Read the model definition and answer for the solid it produces. Units are mm, in the model's axes. A direction names the side the tool comes from. Coordinates: 2 decimals unless noted, no trailing zeros. Loops run counter-clockwise (first coordinate to the right, second up) from the corner with the lowest first, then second, coordinate; pieces in that order, holes last.
from build123d import *

# Parameters (mm, degrees)
SKETCH1_W                             = 70
SKETCH1_H                             = 110
BOTTOM_DEPTH                          = 3.5
SKETCH3_W                             = 70
SKETCH3_H                             = 110
WALL_DEPTH                            = 40
SKETCH4_R                             = 1.625
TOP_PLATE_SCREW_HOLES_DEPTH           = 30
TOP_PLATE_SCREW_HOLES_DRAFT           = -1
TOP_PLATE_SCREW_HOLES_PROFILE_2_DEPTH = 30
TOP_PLATE_SCREW_HOLES_PROFILE_2_DRAFT = -1
TOP_PLATE_SCREW_HOLES_PROFILE_3_DEPTH = 30
TOP_PLATE_SCREW_HOLES_PROFILE_3_DRAFT = -1
TOP_PLATE_SCREW_HOLES_PROFILE_4_DEPTH = 30
TOP_PLATE_SCREW_HOLES_PROFILE_4_DRAFT = -1
FILLET1_R                             = 2
FILLET2_R                             = 2
FILLET3_R                             = 2
FILLET4_R                             = 2
FILLET5_R                             = 2
FILLET6_R                             = 2
FILLET7_R                             = 2
FILLET8_R                             = 2
M4_MOUNT_R                            = 2.1
M4_MOUNT_CUT_DEPTH                    = 77.485292704
CABLE_PASS_CUT_DEPTH                  = 10
SKETCH6_R                             = 1.75
M3_CONNECTION_CUT_DEPTH               = 10


with BuildPart() as part:
    # Sketch1 → Bottom (new body)
    with BuildSketch(Plane(origin=(0, 0, 0), x_dir=(1, 0, 0), z_dir=(0, 1, 0))):
        Rectangle(SKETCH1_W, SKETCH1_H)
    extrude(amount=BOTTOM_DEPTH)

    # Sketch3 → Wall (add)
    with BuildSketch(Plane(origin=(0, 3.5, 0), x_dir=(1, 0, 0), z_dir=(0, 1, 0))):
        Rectangle(SKETCH3_W, SKETCH3_H)
        Polygon((-26, 52), (-4, 52), (26, 52), (26, 46), (32, 46), (32, -46), (26, -46), (26, -52), (4, -52), (-26, -52), (-26, -46), (-32, -46), (-32, 46), (-26, 46), align=None, mode=Mode.SUBTRACT)
    extrude(amount=WALL_DEPTH)


with BuildPart() as top_plate_screw_holes_tool:
    # Sketch4 → Top Plate Screw Holes (with draft: the straight prism first)
    with BuildSketch(Plane(origin=(0, 43.5, 0), x_dir=(1, 0, 0), z_dir=(0, 1, 0))):
        with Locations((-30, 50)):
            Circle(SKETCH4_R)
    extrude(amount=-TOP_PLATE_SCREW_HOLES_DEPTH)
    # Top Plate Screw Holes: the draft: its side faces are tilted about the plane it starts from
    top_plate_screw_holes_sides = [top_plate_screw_holes_tool.faces().sort_by_distance(p)[0] for p in [
        (-31.625, 28.5, -50),
    ]]
    draft(top_plate_screw_holes_sides, Plane(origin=(0, 43.5, 0), x_dir=(1, 0, 0), z_dir=(0, 1, 0)), TOP_PLATE_SCREW_HOLES_DRAFT)


with BuildPart() as part_1:
    add(part.part)

    # Top Plate Screw Holes: cut by top_plate_screw_holes_tool
    add(top_plate_screw_holes_tool.part, mode=Mode.SUBTRACT)


with BuildPart() as top_plate_screw_holes_profile_2_tool:
    # Sketch4 → Top Plate Screw Holes profile 2 (with draft: the straight prism first)
    with BuildSketch(Plane(origin=(0, 43.5, 0), x_dir=(1, 0, 0), z_dir=(0, 1, 0))):
        with Locations((30, 50)):
            Circle(SKETCH4_R)
    extrude(amount=-TOP_PLATE_SCREW_HOLES_PROFILE_2_DEPTH)
    # Top Plate Screw Holes profile 2: the draft: its side faces are tilted about the plane it starts from
    top_plate_screw_holes_profile_2_sides = [top_plate_screw_holes_profile_2_tool.faces().sort_by_distance(p)[0] for p in [
        (28.375, 28.5, -50),
    ]]
    draft(top_plate_screw_holes_profile_2_sides, Plane(origin=(0, 43.5, 0), x_dir=(1, 0, 0), z_dir=(0, 1, 0)), TOP_PLATE_SCREW_HOLES_PROFILE_2_DRAFT)


with BuildPart() as part_2:
    add(part_1.part)

    # Top Plate Screw Holes profile 2: cut by top_plate_screw_holes_profile_2_tool
    add(top_plate_screw_holes_profile_2_tool.part, mode=Mode.SUBTRACT)


with BuildPart() as top_plate_screw_holes_profile_3_tool:
    # Sketch4 → Top Plate Screw Holes profile 3 (with draft: the straight prism first)
    with BuildSketch(Plane(origin=(0, 43.5, 0), x_dir=(1, 0, 0), z_dir=(0, 1, 0))):
        with Locations((30, -50)):
            Circle(SKETCH4_R)
    extrude(amount=-TOP_PLATE_SCREW_HOLES_PROFILE_3_DEPTH)
    # Top Plate Screw Holes profile 3: the draft: its side faces are tilted about the plane it starts from
    top_plate_screw_holes_profile_3_sides = [top_plate_screw_holes_profile_3_tool.faces().sort_by_distance(p)[0] for p in [
        (28.375, 28.5, 50),
    ]]
    draft(top_plate_screw_holes_profile_3_sides, Plane(origin=(0, 43.5, 0), x_dir=(1, 0, 0), z_dir=(0, 1, 0)), TOP_PLATE_SCREW_HOLES_PROFILE_3_DRAFT)


with BuildPart() as part_3:
    add(part_2.part)

    # Top Plate Screw Holes profile 3: cut by top_plate_screw_holes_profile_3_tool
    add(top_plate_screw_holes_profile_3_tool.part, mode=Mode.SUBTRACT)


with BuildPart() as top_plate_screw_holes_profile_4_tool:
    # Sketch4 → Top Plate Screw Holes profile 4 (with draft: the straight prism first)
    with BuildSketch(Plane(origin=(0, 43.5, 0), x_dir=(1, 0, 0), z_dir=(0, 1, 0))):
        with Locations((-30, -50)):
            Circle(SKETCH4_R)
    extrude(amount=-TOP_PLATE_SCREW_HOLES_PROFILE_4_DEPTH)
    # Top Plate Screw Holes profile 4: the draft: its side faces are tilted about the plane it starts from
    top_plate_screw_holes_profile_4_sides = [top_plate_screw_holes_profile_4_tool.faces().sort_by_distance(p)[0] for p in [
        (-31.625, 28.5, 50),
    ]]
    draft(top_plate_screw_holes_profile_4_sides, Plane(origin=(0, 43.5, 0), x_dir=(1, 0, 0), z_dir=(0, 1, 0)), TOP_PLATE_SCREW_HOLES_PROFILE_4_DRAFT)


with BuildPart() as part_4:
    add(part_3.part)

    # Top Plate Screw Holes profile 4: cut by top_plate_screw_holes_profile_4_tool
    add(top_plate_screw_holes_profile_4_tool.part, mode=Mode.SUBTRACT)

    # Fillet1
    fillet1_edges = [part_4.edges().sort_by_distance(p)[0] for p in [
        (-26, 23.5, 46),
    ]]
    fillet(fillet1_edges, radius=FILLET1_R)

    # Fillet2
    fillet2_edges = [part_4.edges().sort_by_distance(p)[0] for p in [
        (26, 23.5, 46),
    ]]
    fillet(fillet2_edges, radius=FILLET2_R)

    # Fillet3
    fillet3_edges = [part_4.edges().sort_by_distance(p)[0] for p in [
        (26, 23.5, -46),
    ]]
    fillet(fillet3_edges, radius=FILLET3_R)

    # Fillet4
    fillet4_edges = [part_4.edges().sort_by_distance(p)[0] for p in [
        (-26, 23.5, -46),
    ]]
    fillet(fillet4_edges, radius=FILLET4_R)

    # Fillet5
    fillet5_edges = [part_4.edges().sort_by_distance(p)[0] for p in [
        (-35, 21.75, -55),
    ]]
    fillet(fillet5_edges, radius=FILLET5_R)

    # Fillet6
    fillet6_edges = [part_4.edges().sort_by_distance(p)[0] for p in [
        (35, 21.75, -55),
    ]]
    fillet(fillet6_edges, radius=FILLET6_R)

    # Fillet7
    fillet7_edges = [part_4.edges().sort_by_distance(p)[0] for p in [
        (35, 21.75, 55),
    ]]
    fillet(fillet7_edges, radius=FILLET7_R)

    # Fillet8
    fillet8_edges = [part_4.edges().sort_by_distance(p)[0] for p in [
        (-35, 21.75, 55),
    ]]
    fillet(fillet8_edges, radius=FILLET8_R)

    # M4 Mount → M4 Mount Cut (cut, through all)
    with BuildSketch(Plane.XZ.offset(-3.5)):
        with Locations(Location((0, -20, 0), (0, 0, 270))):
            Circle(M4_MOUNT_R)
        with Locations(Location((0, 20, 0), (0, 0, 270))):
            Circle(M4_MOUNT_R)
    extrude(amount=M4_MOUNT_CUT_DEPTH, mode=Mode.SUBTRACT)

    # M4 Screw CUT cone 1 section (through the dimple's axis) → M4 Screw CUT (revolve, cut)
    with BuildSketch(Plane(origin=(0, 3.5, 20), x_dir=(0, 0, 1), z_dir=(1, 0, 0))):
        Polygon((0, 0), (3.75, 0), (0, 3.75), align=None)
    revolve(axis=Axis((0, 3.5, 20), (0, -1, 0)), mode=Mode.SUBTRACT)

    # M4 Screw CUT cone 2 section (through the dimple's axis) → M4 Screw CUT cone 2 (revolve, cut)
    with BuildSketch(Plane(origin=(0, 3.5, -20), x_dir=(0, 0, 1), z_dir=(1, 0, 0))):
        Polygon((0, 0), (3.75, 0), (0, 3.75), align=None)
    revolve(axis=Axis((0, 3.5, -20), (0, -1, 0)), mode=Mode.SUBTRACT)

    # Sketch5 → Cable Pass CUT (cut)
    with BuildSketch(Plane.ZY.offset(-32)):
        with BuildLine():
            Line((-46, 3.5), (-34, 3.5))
            add(Edge.make_bspline(
                [(-34, 3.5), (-34, 6.5), (-40, 6.5), (-46, 6.5), (-46, 3.5)],
                knots=[0, 0, 0, 1.570796327, 1.570796327, 3.141592654, 3.141592654, 3.141592654], degree=2, weights=[1, 0.707106781, 1, 0.707106781, 1]))
        make_face()
    extrude(amount=-CABLE_PASS_CUT_DEPTH, mode=Mode.SUBTRACT)

    # Sketch6 → M3 Connection CUT (cut)
    with BuildSketch(Plane.ZY.offset(-32)):
        with Locations((-25, 28.5)):
            Circle(SKETCH6_R)
        with Locations((25, 28.5)):
            Circle(SKETCH6_R)
        with Locations((0, 8.5)):
            Circle(SKETCH6_R)
    extrude(amount=-M3_CONNECTION_CUT_DEPTH, mode=Mode.SUBTRACT)


solid = part_4.part
Item 1: Find the intervals of material crossed by line 1 along Z through (x, y) = (-13, 37); line 2 along X through (y, z) = (7, 1); line 3 along Z through (x, y) = (0, 1), in increasing order.
Numbers:
line 1: z = -55 to -52, 52 to 55
line 2: x = -35 to -32, 32 to 35
line 3: z = -55 to -22.1, -17.9 to 17.9, 22.1 to 55
Item 2: A cutting plane is placed at B-B on y = 8.5. Determine the outline of the cut face in (x, z), then the cut area to 3 significant figures.
Numbers:
outline: (-35, -53) arc R2 ccw to (-33, -55) - (33, -55) arc R2 ccw to (35, -53) - (35, -1.75) - (32, -1.75) - (32, -46) - (28, -46) arc R2 ccw to (26, -48) - (26, -52) - (-26, -52) - (-26, -48) arc R2 ccw to (-28, -46) - (-32, -46) - (-32, 46) - (-28, 46) arc R2 ccw to (-26, 48) - (-26, 52) - (26, 52) - (26, 48) arc R2 ccw to (28, 46) - (32, 46) - (32, 1.75) - (35, 1.75) - (35, 53) arc R2 ccw to (33, 55) - (-33, 55) arc R2 ccw to (-35, 53) - close
area: 1,170 mm2
Item 3: Given pin 1 (3 mm diameter, centred on y = 28.5, z = 25, fed in from +X); pin 2 (20 mm diameter, centred on x = -10.5, z = 5, fed in from +Y); pin 3 (1.8 mm diameter, centred on x = -30, z = -50, fed in from +Y); pin 4 (3.5 mm diameter, centred on x = 0, z = 20, fed in from +Y), each flat-ended and moving along its own axis, determine where each tip first touches the part or whether it passes through.
Numbers:
pin 1: stops at x = -32
pin 2: stops at y = 3.5
pin 3: stops at y = 13.5
pin 4: passes through
Item 4: Determine the mould class of faces 1 (the face through (33.48, 28.58, 23.25)), 2 (the face through (30, 23, 46)), 3 (the face through (-31.366, 28.71, 49.94)) for opening direction Y: released by +Y, released by -Y, zero draft, split by the parting line, or undercut.
Numbers:
face 1: undercut
face 2: zero draft
face 3: released by +Y
Item 5: Which of the six approach directions +Z, -Z, +X, -X, +Y, -Y give full straight-line access (tool end or side, diameter ignored) to faces 4 (the face through (28.634, 28.71, -50.06)), 5 (the face through (-34, 43.5, 4))?
Numbers:
face 4: +Y
face 5: +Z, -Z, +X, -X, +Y
Item 6: A cutting plane is placed at D-D on y = 40. Determine the outline of the cut face in (x, z), then the cut area to 3 significant figures.
Numbers:
outline: (-35, -53) arc R2 ccw to (-33, -55) - (33, -55) arc R2 ccw to (35, -53) - (35, 53) arc R2 ccw to (33, 55) - (-33, 55) arc R2 ccw to (-35, 53) - close; hole (-32, -46) - (-28, -46) arc R2 cw to (-26, -48) - (-26, -52) - (26, -52) - (26, -48) arc R2 cw to (28, -46) - (32, -46) - (32, 46) - (28, 46) arc R2 cw to (26, 48) - (26, 52) - (-26, 52) - (-26, 48) arc R2 cw to (-28, 46) - (-32, 46) - close; hole circle Ø3.13 at (-30, -50); hole circle Ø3.13 at (-30, 50); hole circle Ø3.13 at (30, -50); hole circle Ø3.13 at (30, 50)
area: 1,150 mm2
Item 7: A cutting plane is placed at C-C on x = -11.5. Determine the outline of the cut face in (y, z).
Numbers:
outline: (0, -55) - (43.5, -55) - (43.5, -52) - (3.5, -52) - (3.5, 52) - (43.5, 52) - (43.5, 55) - (0, 55) - close
Item 8: A cutting plane is placed at A-A on z = 25. Determine the outline of the cut face in (x, y), then the cut area to 4 significant figures.
Numbers:
outline: (-35, 0) - (35, 0) - (35, 26.75) - (32, 26.75) - (32, 3.5) - (-32, 3.5) - (-32, 43.5) - (-35, 43.5) - close; (32, 30.25) - (35, 30.25) - (35, 43.5) - (32, 43.5) - close
area: 474.5 mm2
